Geometry: final body of the model. Coordinates: model frame, mm. Face numbers are marked on the shaded views. Give positions to 0.01 mm unless a question says otherwise; leave off trailing zeros. Loops run counter-clockwise (first coordinate to the right, second up) from the corner with the lowest first, then second, coordinate; pieces in that order, holes last.
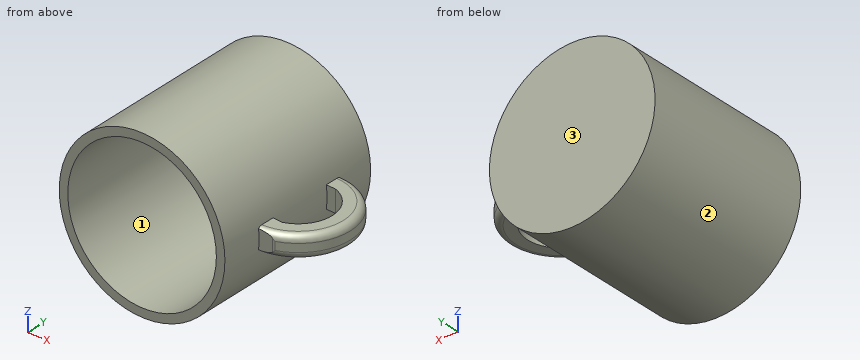
from build123d import *

# Parameters (mm, degrees)
F0_R         = 61.5738591245
F1_DEPTH     = 130.302
F2_T         = -6.35
F4_DEPTH     = 8.128
F5_T1_DEPTH  = 20.8040228352
F5_T3_DEPTH  = 20.562657233
F5_T8_ANGLE  = 182.1562701249
F5_S9_R      = 61.5738591245
F5_T10_DEPTH = 49
F5_T14_ANGLE = 182.1562701249
F5_S15_R     = 61.5738591245
F5_T16_DEPTH = 49


# Not quite as in the source:
# - a fillet or chamfer that OpenCascade refuses, or shapes differently, is made with other operations: its cross-section is extruded or revolved along the edge and cut away or added


with BuildPart() as f1:
    # F0 (on Front) → F1 (new body)
    with BuildSketch(Plane.XZ):
        Circle(F0_R)
    extrude(amount=F1_DEPTH)

    # F2
    f2_openings = [f1.faces().sort_by_distance(p)[0] for p in [
        (0, -130.302, 0),
    ]]
    offset(amount=F2_T, openings=f2_openings)

    # F3 (on Top) → F4 (join, symmetric)
    with BuildSketch(Plane.XY):
        with BuildLine():
            Line((59.0887926519, -99.7823445332), (72.4941612439, -99.7823445332))
            ThreePointArc((72.4941612439, -99.7823445332), (98.9458486723, -62.8559772667), (71.8830453985, -26.3751186382))
            Line((71.8830453985, -26.3751186382), (59.0614564717, -26.3751186382))
            Line((59.0614564717, -26.3751186382), (59.0614564717, -38.9808338419))
            Line((59.0614564717, -38.9808338419), (67.8895905633, -39.1665116223))
            ThreePointArc((67.8895905633, -39.1665116223), (85.5460362932, -62.9675308307), (68.2882977353, -87.0592109513))
            Line((68.2882977353, -87.0592109513), (59.0887926519, -86.546982936))
            Line((59.0887926519, -86.546982936), (59.0887926519, -99.7823445332))
        make_face()
    extrude(amount=F4_DEPTH, both=True)

    # F5: fillet of radius 5.08 on 4 edges, made by hand

    # F5_s2 → F5_t1 (cut)
    with BuildSketch(Plane.XY.offset(-10.4020114176)):
        with BuildLine():
            ThreePointArc((71.6465994249, -99.7823445332), (72.5131887158, -99.7078837649), (73.3543737137, -99.4866842973))
            ThreePointArc((73.3543737137, -99.4866842973), (72.925139457, -99.6370514033), (72.4941612439, -99.7823445332))
            Line((72.4941612439, -99.7823445332), (71.6465994249, -99.7823445332))
        make_face()
    extrude(amount=F5_T1_DEPTH, mode=Mode.SUBTRACT)

    # F5_s4 → F5_t3 (cut)
    with BuildSketch(Plane.XY.offset(-10.2813286165)):
        with BuildLine():
            ThreePointArc((71.0804640636, -26.3751186382), (71.9022151056, -26.4420232646), (72.7023208932, -26.6409748489))
            ThreePointArc((72.7023208932, -26.6409748489), (72.2934256102, -26.5057587291), (71.8830453985, -26.3751186382))
            Line((71.8830453985, -26.3751186382), (71.0804640636, -26.3751186382))
        make_face()
    extrude(amount=F5_T3_DEPTH, mode=Mode.SUBTRACT)


with BuildPart() as f5_tool6:
    # F5_s7 → F5_t8 (revolve)
    with BuildSketch(Plane(origin=(61.0497406785, -0.6405689566, 0), x_dir=(0, 0, 1), z_dir=(-0.9999449575, 0.010491997, 0))):
        with BuildLine():
            ThreePointArc((-8.128, -96.0134100137), (-6.6401024484, -99.6055124621), (-3.048, -101.0934100137))
            Line((-3.048, -101.0934100137), (-8.128, -101.0934100137))
            Line((-8.128, -101.0934100137), (-8.128, -96.0134100137))
        make_face()
    revolve(axis=Axis((60.393573296, -63.1769253215, -8.128), (0, 0, 1)), revolution_arc=F5_T8_ANGLE)

    # F5_s9 → F5_t10 (cut, symmetric)
    with BuildSketch(Plane.XZ.offset(63.2)):
        Circle(F5_S9_R)
    extrude(amount=F5_T10_DEPTH, both=True, mode=Mode.SUBTRACT)


with BuildPart() as f1_1:
    add(f1.part)

    # F5_t5: cut F5_tool6
    add(f5_tool6.part, mode=Mode.SUBTRACT)


with BuildPart() as f5_tool12:
    # F5_s13 → F5_t14 (revolve)
    with BuildSketch(Plane(origin=(61.0497406785, -0.6405689566, 0), x_dir=(0, 0, 1), z_dir=(-0.9999449575, 0.010491997, 0))):
        with BuildLine():
            ThreePointArc((8.128, -96.0134100137), (6.6401024484, -99.6055124621), (3.048, -101.0934100137))
            Line((3.048, -101.0934100137), (8.128, -101.0934100137))
            Line((8.128, -101.0934100137), (8.128, -96.0134100137))
        make_face()
    revolve(axis=Axis((60.393573296, -63.1769253215, 8.128), (0, 0, 1)), revolution_arc=F5_T14_ANGLE)

    # F5_s15 → F5_t16 (cut, symmetric)
    with BuildSketch(Plane.XZ.offset(63.2)):
        Circle(F5_S15_R)
    extrude(amount=F5_T16_DEPTH, both=True, mode=Mode.SUBTRACT)


with BuildPart() as f1_2:
    add(f1_1.part)

    # F5_t11: cut F5_tool12
    add(f5_tool12.part, mode=Mode.SUBTRACT)


solid = f1_2.part
Item 1: Section query C-C on y = -17. Return loops of the section in (x, z).
Values follow:
outline: circle Ø123.15 at (0, 0); hole circle Ø110.45 at (0, 0)
Item 2: Ray query, probe 1 along Z at (x, y) = (0, -31.5); probe 2 along X at (y, z) = (-61, 1.5); probe 3 along Y at (x, z) = (14.5, 33). Return the intervals inside material, ascending.
Values follow:
probe 1: z = -61.57 to -55.22, 55.22 to 61.57
probe 2: x = -61.56 to -55.2, 55.2 to 61.56, 85.45 to 98.89
probe 3: y = -6.35 to 0
Item 3: Section query B-B on z = -15. Return loops of the section in (x, y), plus the area to 3 significant figures.
Values follow:
outline: (-59.72, -130.3) - (-53.15, -130.3) - (-53.15, -6.35) - (53.15, -6.35) - (53.15, -130.3) - (59.72, -130.3) - (59.72, 0) - (-59.72, 0) - close
area: 2,390 mm2
Item 4: Pin query (flat end, axial travel): pin 1 (2 mm diameter, centred on x = 42, y = -81, fed in from +Z); pin 2 (3 mm diameter, centred on x = 64.5, z = -0.5, fed in from -Y); pin 3 (5 mm diameter, centred on x = 65, z = -3.5, fed in from +Y). Return the tip coordinate at first contact, or that it passes through.
Values follow:
pin 1: stops at z = 45.94
pin 2: stops at y = -99.78
pin 3: stops at y = -26.38
Item 5: Section query A-A on x = 0. Return loops of the section in (y, z).
Values follow:
outline: (-130.3, -61.57) - (0, -61.57) - (0, 61.57) - (-130.3, 61.57) - (-130.3, 55.22) - (-6.35, 55.22) - (-6.35, -55.22) - (-130.3, -55.22) - close
Item 6: Draft query along Z for the marked faces 1, 2 and 3. Return one class per face: +Z half, -Z half, draft (parallel to the pull), parting line (faces both ways), or undercut.
Values follow:
face 1: undercut
face 2: parting line
face 3: draft
Item 7: Section query D-D on z = 0. Return loops of the section in (x, y).
Values follow:
outline: (-61.57, -130.3) - (-55.22, -130.3) - (-55.22, -6.35) - (55.22, -6.35) - (55.22, -130.3) - (61.57, -130.3) - (61.57, -99.78) - (71.65, -99.78) arc R5.08 ccw to (73.35, -99.49) arc R38.55 ccw to (72.7, -26.64) arc R5.08 ccw to (71.08, -26.38) - (61.57, -26.38) - (61.57, 0) - (-61.57, 0) - close; hole (61.57, -86.69) - (68.29, -87.06) arc R25.15 ccw to (67.89, -39.17) - (61.57, -39.03) - close
